Autodesk Inventor part; units mm, degrees
ref_plane "YZ Plane" through (0, 0, 0) normal (1, 0, 0) x (0, 1, 0)
ref_plane "XZ Plane" through (0, 0, 0) normal (0, 1, 0) x (-1, 0, 0)
ref_plane "XY Plane" through (0, 0, 0) normal (0, 0, 1) x (1, 0, 0)
sketch "Эскиз3" plane through (0, 0, 0) normal (1, 0, 0) x (0, 1, 0)
  line L0 (0, 0) -> (20, 0)
  line L1 (20, 0) -> (20, 20)
  line L2 (20, 20) -> (0, 20)
  line L3 (0, 20) -> (0, 0)
  line L4 (18.5, 18.5) -> (1.5, 18.5)
  line L5 (1.5, 18.5) -> (1.5, 1.5)
  line L6 (1.5, 1.5) -> (18.5, 1.5)
  line L7 (18.5, 1.5) -> (18.5, 18.5)
  point P0 (10, 18.5)
  point P1 (10, 20)
  point P2 (1.5, 10)
  point P3 (0, 10)
  dimension "d2" = 20
  dimension "d3" = 1.5
extrude "Выдавливание1" add sketch "Эскиз3" along normal blind 50 and the other way blind 30
sketch "Эскиз1" plane through (0, 0, 0) normal (0, 0, 1) x (1, 0, 0)
  circle A0 centre (15, 10) radius 2.5
  circle A1 centre (5, 10) radius 2.5
  point P0 (0, 0)
extrude "Выдавливание2" cut sketch "Эскиз1" along normal through all
sketch "Эскиз4" plane through (-30, 20, 20) normal (0, 1, 0) x (1, 0, 0)
  circle A0 centre (6, 10) radius 2
  circle A1 centre (74, 10) radius 2
  line L0 (80, 20) -> (80, 0) construction
  line L1 (80, 20) -> (0, 20) construction
  line L2 (0, 0) -> (0, 20) construction
  point P0 (30, 20)
  point P1 (80, 10)
  dimension "d10" = 4
  dimension "d11" = 6
  dimension "d12" = 6
extrude "Выдавливание3" cut sketch "Эскиз4" against normal through all
properties part number "2" material "Алюминий 6061"
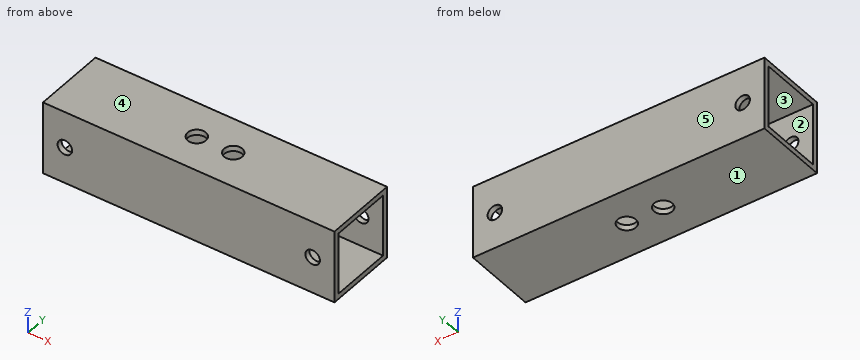
Model file for the job. Use its own axes, mm. Face numbers are marked on the shaded views. A direction names the side the tool comes from. Round coordinates to 2 decimals unless told otherwise and drop trailing zeros. Write each loop counter-clockwise with the first axis right and the second up, starting at its lowest first coordinate (ties: lowest second). Pieces come first, ordered by that corner, then holes. Notation, with made-up numbers: (-5, 32.5) - (0, 32.5) arc R27 ccw to (0, 55.5) - close; hole circle Ø11 at (60.25, 36). An arc over 180 degrees is marked (long way). One line per item, written item: value.
(1) Two-plate mould, pull along Y, no slides. Class the marked faces 3, 4 and 5: pulls with the +Y half, pulls with the -Y half, needs draft (parallel to the pull), parting line crosses it, or undercut.
Values follow:
face 3: undercut
face 4: needs draft
face 5: pulls with the +Y half
(2) Cut at A-A, the plane x = 44. Give the cut face in (y, z), plus the area to 3 significant figures.
Values follow:
outline: (0, 0) - (20, 0) - (20, 8) - (18.5, 8) - (18.5, 1.5) - (1.5, 1.5) - (1.5, 8) - (0, 8) - close; (0, 12) - (1.5, 12) - (1.5, 18.5) - (18.5, 18.5) - (18.5, 12) - (20, 12) - (20, 20) - (0, 20) - close
area: 99.0 mm²
(3) 3-axis set-ups, long thin cutter, end or side, ignore diameter. For the marked faces 1 and 2: which of +Z, -Z, +X, -X, +Y, -Y reach the whole face in a straight line?
Values follow:
face 1: -Z, +X, -X, +Y, -Y
face 2: +X, -X
(4) Wall check: probe 1 along X at (y, z) = (1.15, 10); probe 2 along Z at (x, y) = (32, 17.5); probe 3 along Y at (x, z) = (5, 0.7). Give the ranges that are in metal, low to high.
Values follow:
probe 1: x = -30 to -26, -22 to 42, 46 to 50
probe 2: z = 0 to 1.5, 18.5 to 20
probe 3: y = 0 to 7.5, 12.5 to 20
(5) Drop a flat-ended pin along its axis: P1, Ø5, axis at x = -2, z = 12.5, coming from the -Y side. Give the stop position or say it passes through.
Values follow:
P1: stops at y = 0
(6) Cut at B-B, the plane y = 15. Give the cut face in (x, z).
Values follow:
outline: (-30, 0) - (50, 0) - (50, 1.5) - (-30, 1.5) - close; (-30, 18.5) - (50, 18.5) - (50, 20) - (-30, 20) - close
(7) Cut at D-D, the plane x = 8.5. Give the cut face in (y, z).
Values follow:
outline: (0, 0) - (20, 0) - (20, 20) - (0, 20) - close; hole (1.5, 1.5) - (18.5, 1.5) - (18.5, 18.5) - (1.5, 18.5) - close
